Read the model definition and answer for the solid it produces. Units are mm, in the model's axes. A direction names the side the tool comes from. Give positions to 0.01 mm unless a question says otherwise; leave off trailing zeros. Loops run counter-clockwise (first coordinate to the right, second up) from the corner with the lowest first, then second, coordinate; pieces in that order, holes last. Notation, with made-up numbers: (22.25, 87.5) - (74.25, 87.5) arc R19 cw to (74.25, 119.5) - close; hole circle Ø1 at (-18.5, 0.5). An arc over 180 degrees is marked (long way). Use a Markdown table: item, result. Add a question column.
Item 1: A cutting plane is placed at B-B (z = 24.25). Determine the outline of the cut face in (x, y), plus the area to 3 significant figures.
Item 2: Which of the six approach directions +Z, -Z, +X, -X, +Y, -Y give full straight-line access (tool end or side, diameter ignored) to faces 1 (the face through (5.891, -48, 14)), 2 (the face through (3.391, -51, 14)), 3 (the face through (6.6, -63.5, 19.4))?
Item 3: A cutting plane is placed at D-D (y = -71). Determine the outline of the cut face in (x, z).
Item 4: Each of these flat-tipped pins is pushed along its axis until it touches: P1, Ø3, axis at x = 17, z = 9, coming from the +Y side; P2, Ø4.5, axis at x = 12, y = -44, coming from the +Z side; P3, Ø6.5, axis at y = -51, z = 9.5, coming from the +X side. Where does it stop, or does it pass through?
Item 5: A cutting plane is placed at C-C (y = -45.5). Determine the outline of the cut face in (x, z).
Item 6: Consider probe 1 along Z at (x, y) = (20.5, -53); probe 2 along Z at (x, y) = (12, -19.5); probe 3 along X at (y, z) = (-28.5, 22.25). Determine where each line is inside the solid, lowest interval first. Write a range as [from, to].
Item 7: A cutting plane is placed at A-A (y = -21). Determine the outline of the cut face in (x, z).
from build123d import *

# Parameters (mm, degrees)
F0_W     = 26.8478
F0_H     = 28.7274
F1_DEPTH = 38.1
F2_W     = 20.0660005145
F2_H     = 21.9456005145
F3_DEPTH = 25.4
F5_DEPTH = 19.05
F6_R     = 7.62
F7_T     = -2.5


with BuildPart() as f1:
    # F0 (on Front) → F1 (new body)
    with BuildSketch(Plane.XZ):
        with Locations((13.4239, 14.3637)):
            Rectangle(F0_W, F0_H)
    extrude(amount=F1_DEPTH)

    # F2 (on face) → F3 (join)
    with BuildSketch(Plane.XZ.offset(38.1)):
        with Locations((13.4239, 14.3637)):
            Rectangle(F2_W, F2_H)
    extrude(amount=F3_DEPTH)

    # F4 (on face) → F5 (join)
    with BuildSketch(Plane.XZ.offset(63.5)):
        with BuildLine():
            ThreePointArc((21.7445834799, 14.3637), (19.3075117128, 20.2473117128), (13.4239, 22.6843834799))
            ThreePointArc((13.4239, 22.6843834799), (7.5402882872, 8.4800882872), (21.7445834799, 14.3637))
        make_face()
    extrude(amount=F5_DEPTH)

    # F6
    f6_edges = [f1.edges().sort_by_distance(p)[0] for p in [
        (5.103217, -82.55, 14.3637),
    ]]
    fillet(f6_edges, radius=F6_R)

    # F7
    f7_openings = [f1.faces().sort_by_distance(p)[0] for p in [
        (13.4239, 0, 14.3637),
    ]]
    offset(amount=F7_T, openings=f7_openings, kind=Kind.INTERSECTION)


solid = f1.part
Geometry says:
| question | item | result |
|---|---|---|
| 1 | outline | (0, -38.1) - (3.39, -38.1) - (3.39, -63.5) - (23.46, -63.5) - (23.46, -38.1) - (26.85, -38.1) - (26.85, 0) - (24.35, 0) - (24.35, -35.6) - (2.5, -35.6) - (2.5, 0) - (0, 0) - close |
| 1 | area | 755 mm² |
| 2 | face 1 | +Y |
| 2 | face 2 | +Z, -Z, -X, -Y |
| 2 | face 3 | -Y |
| 3 | outline | circle Ø16.64 at (13.42, 14.36); hole circle Ø11.64 at (13.42, 14.36) |
| 4 | P1 | y = -61 |
| 4 | P2 | z = 25.34 |
| 4 | P3 | x = 23.46 |
| 5 | outline | (3.39, 3.39) - (23.46, 3.39) - (23.46, 25.34) - (3.39, 25.34) - close; hole (5.89, 5.89) - (20.96, 5.89) - (20.96, 22.84) - (5.89, 22.84) - close |
| 6 | probe 1 | [3.39, 5.89], [22.84, 25.34] |
| 6 | probe 2 | [0, 2.5], [26.23, 28.73] |
| 6 | probe 3 | [0, 2.5], [24.35, 26.85] |
| 7 | outline | (0, 0) - (26.85, 0) - (26.85, 28.73) - (0, 28.73) - close; hole (2.5, 2.5) - (24.35, 2.5) - (24.35, 26.23) - (2.5, 26.23) - close |
